Can you work these out from the model? Positions are in its coordinate system, mm. Face numbers are marked on the shaded views. A direction names the side the tool comes from. Give positions to 0.01 mm unless a question says otherwise; leave off trailing zeros. Write each loop counter-clockwise with the first axis right and the second up, starting at its lowest first coordinate (ties: lowest second). Pieces come first, ordered by that corner, then holes. Notation, with made-up numbers: (74.25, 46.25) -> (113.25, 46.25) arc R21 ccw to (113.25, 73.25) -> close; hole circle Ø4 at (23, -6.75). An arc over 180 degrees is marked (long way). One line per item, written item: value.
from build123d import *

# Parameters (mm, degrees)
F0_R     = 3
F0_R_2   = 2.15
F1_DEPTH = 8
F2_W     = 15
F2_H     = 10
F3_DEPTH = 20
F4_R     = 3.25
F6_DEPTH = 18
F7_DEPTH = 5
F8_DEPTH = 8


with BuildPart() as f1:
    # F0 (on Top) → F1 (new body)
    with BuildSketch(Plane.XY):
        Circle(F0_R)
        Circle(F0_R_2, mode=Mode.SUBTRACT)
    extrude(amount=-F1_DEPTH)

    # F2 (on face) → F3 (join)
    with BuildSketch(Plane.XY):
        Rectangle(F2_W, F2_H)
    extrude(amount=F3_DEPTH)

    # F4 (on face) → F6 (cut)
    with BuildSketch(Plane.XY.offset(20)):
        Circle(F4_R)
    extrude(amount=-F6_DEPTH, mode=Mode.SUBTRACT)

    # F5 (on face) → F7 (cut)
    with BuildSketch(Plane.XZ.offset(5)):
        Polygon((-4, 2), (0, 2), (4, 2), (4, 10), (0, 10), (-4, 10), align=None)
    extrude(amount=-F7_DEPTH, mode=Mode.SUBTRACT)

    # F8 (add): a face of the model
    f8_faces = [f1.faces().sort_by_distance(p)[0] for p in [
        (7.3197224362, 0, 0),
    ]]
    extrude(f8_faces, amount=F8_DEPTH)


solid = f1.part
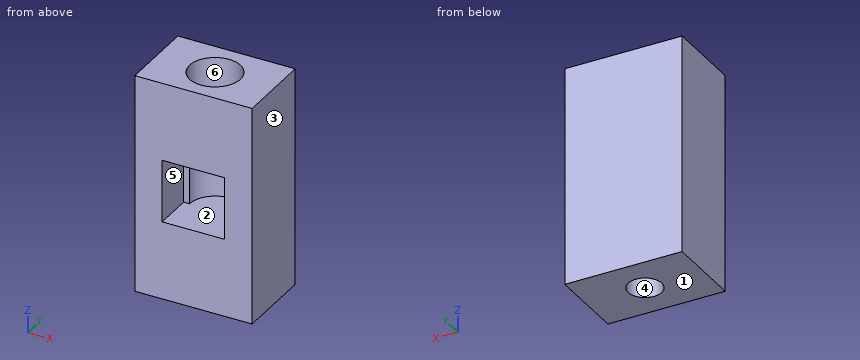
1) For the marked faces 4, 5 and 6, which set-ups out of +Z, -Z, +X, -X, +Y, -Y let a thin tool reach every point of the face, with its end or its side?
Answer list:
face 4: -Z
face 5: -Y
face 6: +Z
2) If we section it at A-A (x = 0): Write out the boundary of the cut face in (y, z), and give its area (3 significant figures).
Answer list:
outline: (-5, -8) -> (-2.15, -8) -> (-2.15, 0) -> (2.15, 0) -> (2.15, -8) -> (5, -8) -> (5, 20) -> (3.25, 20) -> (3.25, 2) -> (-5, 2) -> close; (-5, 10) -> (-3.25, 10) -> (-3.25, 20) -> (-5, 20) -> close
area: 115 mm^2
3) We'd pull the mould along X, two halves only. Please class the marked faces 1, 2 and 3: released by +X, released by -X, zero draft, split by the parting line, or undercut.
Answer list:
face 1: zero draft
face 2: undercut
face 3: released by +X
4) I need wall thicknesses on L1, parallel to Y at x = 0, z = 15.75; L2, parallel to X at y = 0, z = 12.25; L3, parallel to Y at x = 0, z = -4.5. Which ranges of each line are inside material? Lowest first, please.
Answer list:
L1: y = -5 to -3.25, 3.25 to 5
L2: x = -7.5 to -3.25, 3.25 to 7.5
L3: y = -5 to -2.15, 2.15 to 5
5) If we section it at C-C (y = -0.5): Write out the boundary of the cut face in (x, z), and give its area (3 significant figures).
Answer list:
outline: (-7.5, -8) -> (-2.09, -8) -> (-2.09, 0) -> (2.09, 0) -> (2.09, -8) -> (7.5, -8) -> (7.5, 20) -> (3.21, 20) -> (3.21, 10) -> (4, 10) -> (4, 2) -> (-4, 2) -> (-4, 10) -> (-3.21, 10) -> (-3.21, 20) -> (-7.5, 20) -> close
area: 258 mm^2
6) Will these pins go through, and if not, where does the flat tip stop? pin 1 (3.5 mm diameter, centred on x = 0, y = 0, fed in from -Z); pin 2 (1 mm diameter, centred on x = -1.5, y = -1.5, fed in from +Z).
Answer list:
pin 1: stops at z = 0
pin 2: stops at z = 2
7) If we section it at D-D (z = 11): Write out the boundary of the cut face in (x, y), and give its area (3 significant figures).
Answer list:
outline: (-7.5, -5) -> (7.5, -5) -> (7.5, 5) -> (-7.5, 5) -> close; hole circle Ø6.5 at (0, 0)
area: 117 mm^2
8) If we section it at B-B (z = 7): Write out the boundary of the cut face in (x, y).
Answer list:
outline: (-7.5, -5) -> (-4, -5) -> (-4, 0) -> (-3.25, 0) arc R3.25 cw to (3.25, 0) -> (4, 0) -> (4, -5) -> (7.5, -5) -> (7.5, 5) -> (-7.5, 5) -> close
